Part model, mm, in its own coordinate system. A direction names the side the tool comes from. Coordinates: 2 decimals unless noted, no trailing zeros. Order: outer loops, then holes, each group sorted by start corner. A loop starts at its lowest first (then second) coordinate and runs counter-clockwise, first axis right, second up. Notation, with made-up numbers: M 20,84 L 66,84 A25 ccw 66,105 Z; hole C 4.5,5.25 d10. An arc over 180 degrees is marked long. Write item = value, one per line. Start each with the question number.
from build123d import *

# Parameters (mm, degrees)
SKETCH1_R           = 30
BOSS_EXTRUDE1_DEPTH = 26
BOSS_EXTRUDE2_DEPTH = 250
SKETCH4_R           = 13
CUT_EXTRUDE2_DEPTH  = 26
SKETCH1_2_R         = 30
CUT_EXTRUDE3_DEPTH  = 8
SKETCH1_3_R         = 30
CUT_EXTRUDE4_DEPTH  = 8
SKETCH5_R           = 19
CUT_EXTRUDE5_DEPTH  = 210
SKETCH7_W           = 4
SKETCH7_H           = 4
BOSS_EXTRUDE4_DEPTH = 26
SKETCH9_R           = 19
SKETCH9_R_2         = 18
BOSS_EXTRUDE5_DEPTH = 10


with BuildPart() as part:
    # Sketch1 → Boss-Extrude1 (new body, symmetric)
    with BuildSketch(Plane(origin=(0, 0, 0), x_dir=(1, 0, 0), z_dir=(0, 1, 0))):
        Circle(SKETCH1_R)
    extrude(amount=BOSS_EXTRUDE1_DEPTH, both=True)

    # Sketch3 → Boss-Extrude2 (add)
    with BuildSketch(Plane.XY):
        with BuildLine():
            Line((26, 26), (26, 23))
            Line((26, 23), (-2, 23))
            ThreePointArc((-2, 23), (-25, 0), (-2, -23))
            Line((-2, -23), (26, -23))
            Line((26, -23), (26, -26))
            Line((26, -26), (30, -26))
            Line((30, -26), (30, 26))
            Line((30, 26), (26, 26))
        make_face()
    extrude(amount=BOSS_EXTRUDE2_DEPTH)

    # Sketch4 → Cut-Extrude2 (cut, symmetric)
    with BuildSketch(Plane(origin=(0, 0, 0), x_dir=(1, 0, 0), z_dir=(0, 1, 0))):
        Circle(SKETCH4_R)
    extrude(amount=CUT_EXTRUDE2_DEPTH, both=True, mode=Mode.SUBTRACT)

    # Sketch1_2 → Cut-Extrude3 (cut)
    with BuildSketch(Plane(origin=(0, 0, 0), x_dir=(1, 0, 0), z_dir=(0, 1, 0))):
        Circle(SKETCH1_2_R)
    extrude(amount=-CUT_EXTRUDE3_DEPTH, mode=Mode.SUBTRACT)

    # Sketch1_3 → Cut-Extrude4 (cut)
    with BuildSketch(Plane(origin=(0, 0, 0), x_dir=(1, 0, 0), z_dir=(0, 1, 0))):
        Circle(SKETCH1_3_R)
    extrude(amount=CUT_EXTRUDE4_DEPTH, mode=Mode.SUBTRACT)

    # Sketch5 → Cut-Extrude5 (cut)
    with BuildSketch(Plane.XY.offset(250)):
        with Locations((-2, 0)):
            Circle(SKETCH5_R)
    extrude(amount=-CUT_EXTRUDE5_DEPTH, mode=Mode.SUBTRACT)

    # Sketch7 → Boss-Extrude4 (add, symmetric)
    with BuildSketch(Plane(origin=(0, 0, 0), x_dir=(1, 0, 0), z_dir=(0, 1, 0))):
        with Locations((28, -252)):
            Rectangle(SKETCH7_W, SKETCH7_H)
    extrude(amount=BOSS_EXTRUDE4_DEPTH, both=True)

    # Sketch9 → Boss-Extrude5 (add)
    with BuildSketch(Plane.XY.offset(250)):
        with Locations((-2, 0)):
            Circle(SKETCH9_R)
        with Locations((-2, 0)):
            Circle(SKETCH9_R_2, mode=Mode.SUBTRACT)
    extrude(amount=-BOSS_EXTRUDE5_DEPTH)


solid = part.part
Item 1: Flat gauge pins, fed straight in: pin 1 (5 mm diameter, centred on x = 2.5, z = 95, fed in from -Y); pin 2 (8 mm diameter, centred on x = -11.5, z = 207.5, fed in from +Y); pin 3 (6 mm diameter, centred on x = -24, z = 65.5, fed in from -Y). Where does each tip first touch, or does it go through?
Item 2: Cut at C-C, the plane y = -12.5. Write the cut outline in (x, z), and give its area (3 significant figures).
Item 3: Pull direction Z, two halves, no side cores. Call faces 1 (the cylindrical face through (-24.994, 0.506, 131.658)), 2 (the flat face through (17, 0, 250)), 3 (the cylindrical face through (-10.316, 17.126, 7.91)): pulls with the +Z half, pulls with the -Z half, needs draft (parallel to the pull), parting line crosses it, or undercut.
Item 4: Cut at B-B, the plane x = 3. Write the cut outline in (y, z), and give its area (3 significant figures).
Item 5: Wall check: line 1 along Y through (x, z) = (-2, 180); line 2 along X through (y, z) = (18.75, 0); line 3 along Y through (x, z) = (-2, 245). Give the ranges that are in metal, low to high. Write a range as [from, to].
Item 6: 3-axis set-ups, long thin cutter, end or side, ignore diameter. For faces 4 (the cylindrical face through (-4.343, 17.847, 245.07)), 5 (the cylindrical face through (16.12, 5.71, 141.4)), 6 (the flat face through (6, 8, 13)): which of +Z, -Z, +X, -X, +Y, -Y reach the whole face in a straight line?
Item 7: Cut at D-D, the plane z = 8.5. Write the cut outline in (x, y).
Item 8: Cut at A-A, the plane z = 122.5. Write the cut outline in (x, y).
Filled sheet:
q1.pin_1 = -23
q1.pin_2 = 22.33
q1.pin_3 = -12.96
q2.outline = M -21.31,21.12 A30 ccw long 30,0 L 30,254 L 26,254 L 26,250 L 10.95,250 L 10.95,240 L 12.31,240 L 12.31,40 L -16.31,40 L -16.31,240 L -14.95,240 L -14.95,250 L -21.31,250 Z; hole C 0,0 d26
q2.area = 7,870 mm2
q3.face_1 = needs draft
q3.face_2 = pulls with the +Z half
q3.face_3 = undercut
q4.outline = M -26,-29.85 L -8,-29.85 L -8,-12.65 L -26,-12.65 Z; M -26,12.65 L -8,12.65 L -8,29.85 L 8,29.85 L 8,12.65 L 26,12.65 L 26,29.85 L 23,29.85 L 23,250 L 17.29,250 L 17.29,240 L 18.33,240 L 18.33,40 L -18.33,40 L -18.33,240 L -17.29,240 L -17.29,250 L -23,250 L -23,29.85 L -26,29.85 Z; M 8,-29.85 L 26,-29.85 L 26,-12.65 L 8,-12.65 Z
q4.area = 3,690 mm2
q5.line_1 = [-23, -19], [19, 23]
q5.line_2 = [-30, -13], [13, 30]
q5.line_3 = [-23, -18], [18, 23]
q6.face_4 = +Z
q6.face_5 = none
q6.face_6 = -Z
q7.outline = M -28.77,-26 L -9.84,-26 L -9.84,-8 L -28.77,-8 Z; M -28.77,8 L -9.84,8 L -9.84,26 L -28.77,26 Z; M 9.84,-26 L 30,-26 L 30,26 L 9.84,26 L 9.84,8 L 28.77,8 L 28.77,-8 L 9.84,-8 Z
q8.outline = M -2,-23 L 26,-23 L 26,-26 L 30,-26 L 30,26 L 26,26 L 26,23 L -2,23 A23 ccw Z; hole C -2,0 d38
